Geometry: final body of the model. Coordinates: model frame, mm. Face numbers are marked on the shaded views. Give positions to 0.01 mm unless a question says otherwise; leave off trailing zeros. Write each loop counter-clockwise with the first axis right and the second up, starting at its lowest first coordinate (ties: lowest second). Pieces come first, ordered by that corner, then holes.
```python
from build123d import *

# Parameters (mm, degrees)
SKETCH3_R          = 8.2
CUT_EXTRUDE1_DEPTH = 40
CHAMFER1_SIZE      = 1.5
FILLET2_R          = 0.6
FILLET3_R          = 0.6
FILLET4_R          = 0.6


with BuildPart() as part:
    # Sketch2 → Revolve1 (revolve)
    with BuildSketch(Plane(origin=(0, 0, 0), x_dir=(0, 0, -1), z_dir=(1, 0, 0)), mode=Mode.PRIVATE) as revolve1_sk:
        Polygon((-15, 10.2), (-15, 0), (0, 0), (0, 8.2), (20, 19), (20, 21), (0, 10.2), align=None)
    revolve(revolve1_sk.sketch.rotate(Axis((0, 0, 15), (0, 0, -1)), 90), axis=Axis((0, 0, 15), (0, 0, -1)))

    # Sketch3 → Cut-Extrude1 (cut)
    with BuildSketch(Plane.XY.offset(15)):
        Circle(SKETCH3_R)
    extrude(amount=-CUT_EXTRUDE1_DEPTH, mode=Mode.SUBTRACT)

    # Chamfer1
    chamfer1_edges = [part.edges().sort_by_distance(p)[0] for p in [
        (-8.2, 0, 15),
    ]]
    chamfer(chamfer1_edges, length=CHAMFER1_SIZE)

    # Fillet2
    fillet2_edges = [part.edges().sort_by_distance(p)[0] for p in [
        (-21, 0, -20),
        (-19, 0, -20),
    ]]
    fillet(fillet2_edges, radius=FILLET2_R)

    # Fillet3
    fillet3_edges = [part.edges().sort_by_distance(p)[0] for p in [
        (-10.2, 0, 0),
    ]]
    fillet(fillet3_edges, radius=FILLET3_R)

    # Fillet4
    fillet4_edges = [part.edges().sort_by_distance(p)[0] for p in [
        (-8.2, 0, 0),
    ]]
    fillet(fillet4_edges, radius=FILLET4_R)


solid = part.part
```
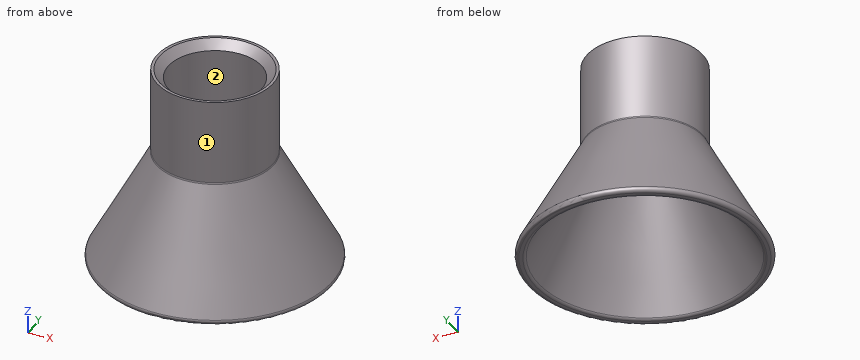
Item 1: Pin query (flat end, axial travel): pin 1 Ø4 at (x, z) = (-0.5, 7) entering from -Y; pin 2 Ø3 at (x, y) = (-14, 10.5) entering from +Z; pin 3 Ø10 at (x, z) = (16, 3.5) entering from -Y; pin 4 Ø5 at (x, y) = (15.5, 8) entering from +Z. Return the tip coordinate at first contact, or that it passes through.
Found:
pin 1: stops at y = -10.2
pin 2: stops at z = -10.74
pin 3: passes through
pin 4: stops at z = -8.78
Item 2: Line query: L1, parallel to Y at x = 0, z = 3; L2, parallel to Y at x = 7, z = 5.5; L3, parallel to X at y = 5, z = -14. Output: solid intervals per line, ascending.
Found:
L1: y = -10.2 to -8.2, 8.2 to 10.2
L2: y = -7.42 to -4.27, 4.27 to 7.42
L3: x = -17.04 to -14.95, 14.95 to 17.04
Item 3: Section B-B, the plane z = 2. Return the cut outline in (x, y).
Found:
outline: circle Ø20.4 at (0, 0); hole circle Ø16.4 at (0, 0)
Item 4: Section A-A, the plane z = -9.5. Return the cut outline in (x, y).
Found:
outline: circle Ø30.66 at (0, 0); hole circle Ø26.66 at (0, 0)
Item 5: Pull-direction query (Y, two-part tool) for the marked faces 1 and 2; classes: +Y half, -Y half, draft (parallel to the pull), parting line (faces both ways), or undercut.
Found:
face 1: parting line
face 2: undercut
